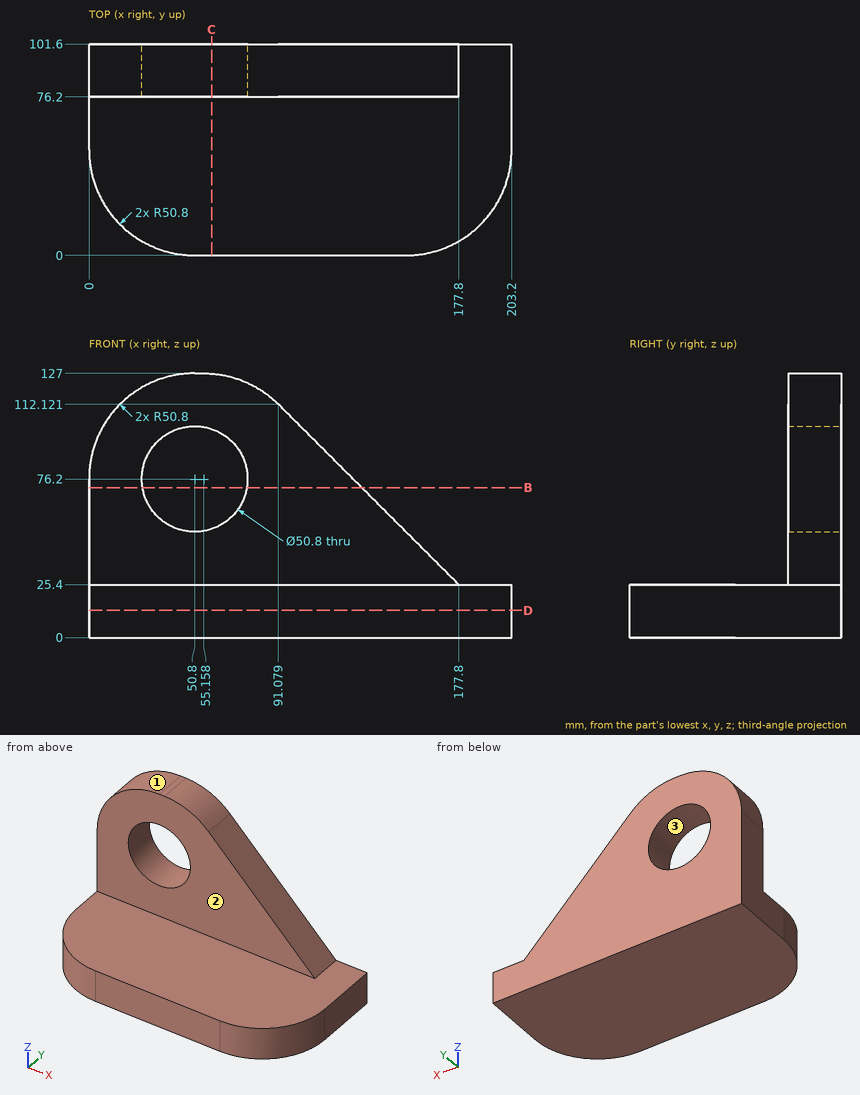
Design review of the part shown in the three views and the two pictorial views. Dimensions are in mm from the part's minimum x, y and z. Round coordinates to 2 decimals unless told otherwise and drop trailing zeros. Loops run counter-clockwise (first coordinate to the right, second up) from the corner with the lowest first, then second, coordinate; pieces in that order, holes last. Notation, with made-up numbers: (52.25, -1.5) - (95.25, -1.5) arc R19 cw to (95.25, 28.5) - close; hole circle Ø3 at (65, 87.25). An arc over 180 degrees is marked (long way). One line per item, written item: value. Start each with the question number.
Item 1: Clearance check with flat-ended pins moving along their axes: pin 1 Ø8 at (x, y) = (117.5, 29.5) entering from +Z; pin 2 Ø2 at (x, y) = (82, 84) entering from +Z. State where each tip first meets the part, or that it passes through.
Item 2: The part is to be moulded in two halves that separate along Z. For the marked faces 1, 2 and 3, say which applies: +Z half, -Z half, draft (parallel to the pull), parting line (faces both ways), or undercut.
Item 3: For L1, parallel to Z at x = 50.8, y = 85; L2, parallel to Y at x = 90, z = 75; L3, parallel to Z at x = 38, y = 47, list the stretches that pass through material, from the lowest coordinate up.
Item 4: Take a section at D-D (z = 13). Give the boundary of the cut face in (x, y), plus the area to 3 significant figures.
Item 5: Take a section at C-C (x = 59). Give the boundary of the cut face in (y, z), plus the area to 3 significant figures.
Item 6: Take a section at B-B (z = 72). Give the boundary of the cut face in (x, y), plus the area to 3 significant figures.
Answer below:
1. pin 1: stops at z = 25.4
1. pin 2: stops at z = 119.94
2. face 1: +Z half
2. face 2: draft
2. face 3: undercut
3. L1: z = 0 to 50.8, 101.6 to 127
3. L2: y = 76.2 to 101.6
3. L3: z = 0 to 25.4
4. outline: (0, 50.8) arc R50.8 ccw to (50.8, 0) - (152.4, 0) arc R50.8 ccw to (203.2, 50.8) - (203.2, 101.6) - (0, 101.6) - close
4. area: 19,500 mm2
5. outline: (0, 0) - (101.6, 0) - (101.6, 52.16) - (76.2, 52.16) - (76.2, 25.4) - (0, 25.4) - close; (76.2, 100.24) - (101.6, 100.24) - (101.6, 126.85) - (76.2, 126.85) - close
5. area: 3,940 mm2
6. outline: (0, 76.2) - (25.75, 76.2) - (25.75, 101.6) - (0, 101.6) - close; (75.85, 76.2) - (131.2, 76.2) - (131.2, 101.6) - (75.85, 101.6) - close
6. area: 2,060 mm2
